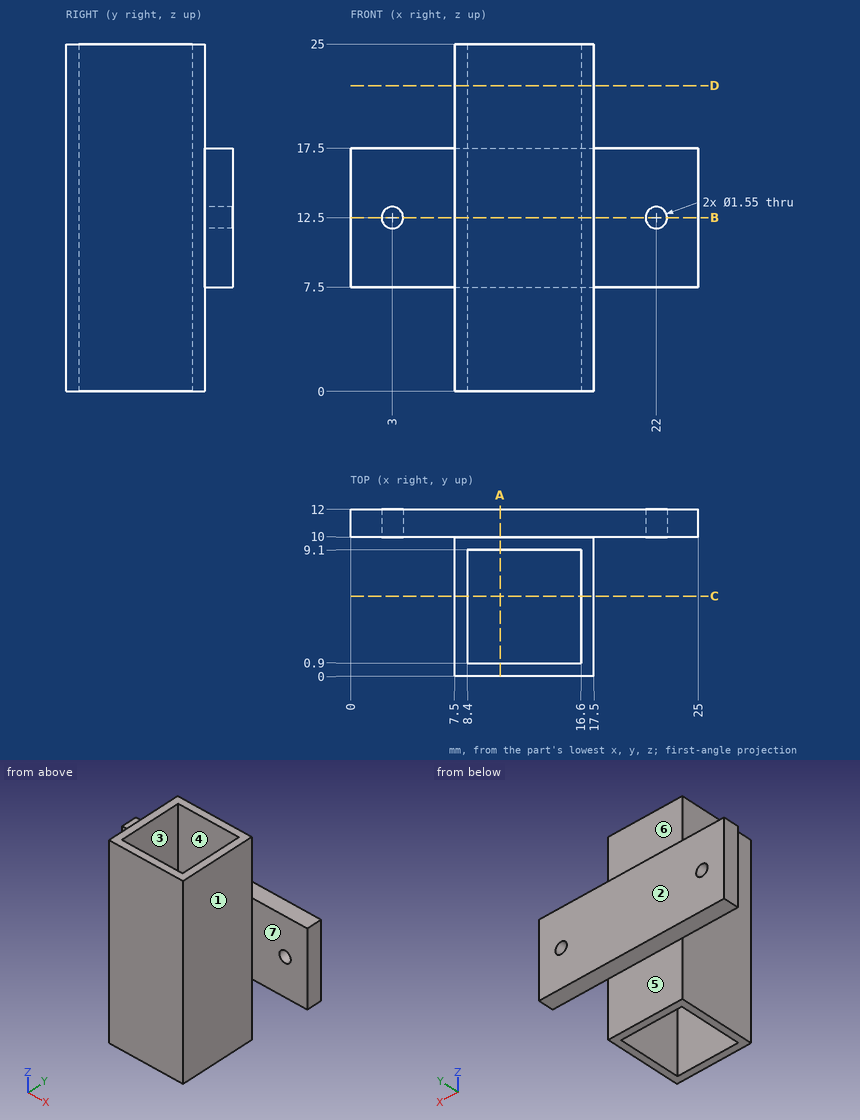
Could you check a few things on this drawing? It's one solid part, dimensions in mm from its lowest x, y, z. A direction names the side the tool comes from. Give positions to 0.01 mm unless a question says otherwise; leave off trailing zeros. Order: outer loops, then holes, each group sorted by start corner. A loop starts at its lowest first (then second) coordinate and runs counter-clockwise, first axis right, second up. Notation, with made-up numbers: (14, -14.75) - (61, -14.75) arc R22 cw to (61, 21.25) - close; hole circle Ø1 at (-3.5, -7). An arc over 180 degrees is marked (long way). One line per item, written item: value. Start each with the question number.
1. Thinking about a two-plate mould opening in X: for the marked faces 1, 2 and 3, which applies, +X half, -X half, draft (parallel to the pull), parting line (faces both ways), or undercut?
2. For the marked faces 4, 5, 6 and 7, which set-ups out of +Z, -Z, +X, -X, +Y, -Y let a thin tool reach every point of the face, with its end or its side?
3. Imagine slicing it at C-C on y = 5.75. List the corners of the cut face in (x, z) for me, plus the area to 3 significant figures.
4. Imagine slicing it at D-D on z = 22. List the corners of the cut face in (x, y) for me, plus the area to 3 significant figures.
5. Imagine slicing it at A-A on x = 10.75. List the corners of the cut face in (y, z) for me.
6. For P1, Ø1.6, axis at x = 14, y = 11, coming from the +Z side; P2, Ø4, axis at x = 3.5, z = 14.5, coming from the -Y side; P3, Ø4, axis at y = 10.5, z = 18.5, coming from the +X side; P4, Ø6.5, axis at y = 3, z = 11.5, coming from the -X side, each with a flat end and sliding along its axis, tell me the tip position at first contact or that it passes through.
7. Imagine slicing it at B-B on z = 12.5. List the corners of the cut face in (x, y) for me (3 decimals).
8. If I drill on probe 1 along X at (y, z) = (11.25, 12.5) (3 decimals); probe 2 along X at (y, z) = (7, 7.5); probe 3 along Z at (x, y) = (22, 10.5) (3 decimals), over which ranges is the centre line in solid material (lowest first)?
Values:
1. face 1: +X half
1. face 2: draft
1. face 3: undercut
2. face 4: +Z, -Z
2. face 5: -Z, +X, -X, +Y
2. face 6: +Z, +X, -X, +Y
2. face 7: +Z, -Z, +X, -Y
3. outline: (7.5, 0) - (8.4, 0) - (8.4, 25) - (7.5, 25) - close; (16.6, 0) - (17.5, 0) - (17.5, 25) - (16.6, 25) - close
3. area: 45.0 mm²
4. outline: (7.5, 0) - (17.5, 0) - (17.5, 10) - (7.5, 10) - close; hole (8.4, 0.9) - (16.6, 0.9) - (16.6, 9.1) - (8.4, 9.1) - close
4. area: 32.8 mm²
5. outline: (0, 0) - (0.9, 0) - (0.9, 25) - (0, 25) - close; (9.1, 0) - (10, 0) - (10, 7.5) - (12, 7.5) - (12, 17.5) - (10, 17.5) - (10, 25) - (9.1, 25) - close
6. P1: z = 17.5
6. P2: y = 10
6. P3: x = 25
6. P4: x = 7.5
7. outline: (0, 10) - (2.225, 10) - (2.225, 12) - (0, 12) - close; (3.775, 10) - (7.5, 10) - (7.5, 0) - (17.5, 0) - (17.5, 10) - (21.225, 10) - (21.225, 12) - (3.775, 12) - close; (22.775, 10) - (25, 10) - (25, 12) - (22.775, 12) - close; hole (8.4, 0.9) - (16.6, 0.9) - (16.6, 9.1) - (8.4, 9.1) - close
8. probe 1: 0 to 2.225, 3.775 to 21.225, 22.775 to 25
8. probe 2: 7.5 to 8.4, 16.6 to 17.5
8. probe 3: 7.5 to 11.725, 13.275 to 17.5
